Can you work these out from the drawing? Everything is in mm from the part's minimum corner. Round coordinates to 2 decimals unless told otherwise and drop trailing zeros. Order: outer loops, then holes, each group sorted by start corner. A loop starts at its lowest first (then second) coordinate and runs counter-clockwise, first axis right, second up. Notation, with made-up numbers: (14, 7) - (48, 7) arc R26 ccw to (48, 27) - close; hole circle Ø8 at (23.5, 77). An arc over 180 degrees is marked (long way). Answer as a JSON object with one key per item and string values.
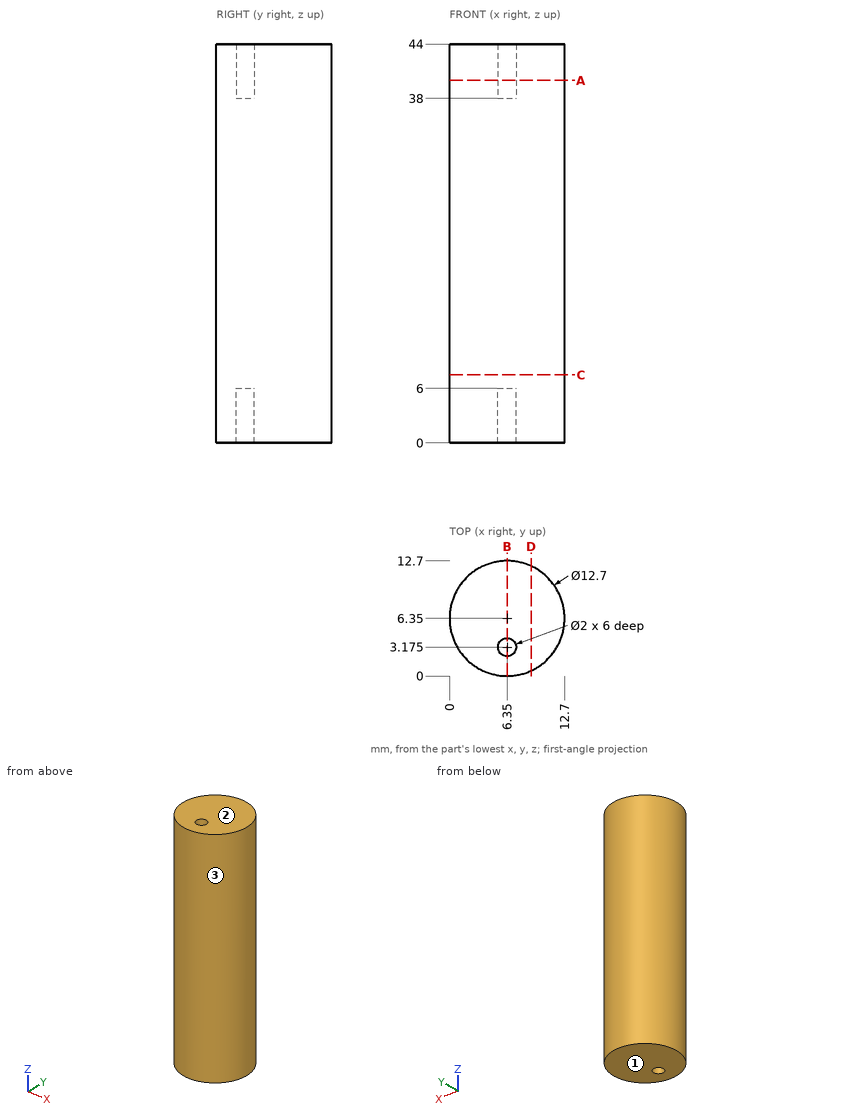
1. For P1, Ø1, axis at x = 9, y = 3.5, coming from the -Z side; P2, Ø6, axis at y = 11, z = 24, coming from the -X side; P3, Ø4, axis at x = 11.5, z = 36, coming from the +Y side; P4, Ø1.5, axis at x = 4.5, z = 31, coming from the +Y side, each with a flat end and sliding along its axis, tell me the tip position at first contact or that it passes through.
Responses:
{"P1": "z = 0", "P2": "x = 0.22", "P3": "y = 11.86", "P4": "y = 12.6"}
2. Thinking about a two-plate mould opening in Z: for the marked faces 1, 2 and 3, which applies, pulls with the +Z half, pulls with the -Z half, needs draft (parallel to the pull), parting line crosses it, or undercut?
Responses:
{"face 1": "pulls with the -Z half", "face 2": "pulls with the +Z half", "face 3": "needs draft"}
3. Imagine slicing it at A-A (z = 40). List the corners of the cut face in (x, y) for me (3 decimals), plus the area to 3 significant figures.
Responses:
{"outline": "circle Ø12.7 at (6.35, 6.35); hole circle Ø2 at (6.35, 3.175)", "area": "124 mm2"}
4. Imagine slicing it at D-D (x = 9). List the corners of the cut face in (y, z) for me.
Responses:
{"outline": "(0.58, 0) - (12.12, 0) - (12.12, 44) - (0.58, 44) - close"}
5. Imagine slicing it at B-B (x = 6.35). List the corners of the cut face in (y, z) for me (3 decimals), plus the area to 3 significant figures.
Responses:
{"outline": "(0, 0) - (2.175, 0) - (2.175, 6) - (4.175, 6) - (4.175, 0) - (12.7, 0) - (12.7, 44) - (4.175, 44) - (4.175, 38) - (2.175, 38) - (2.175, 44) - (0, 44) - close", "area": "535 mm2"}
6. Imagine slicing it at C-C (z = 7.5). List the corners of the cut face in (x, y) for me.
Responses:
{"outline": "circle Ø12.7 at (6.35, 6.35)"}
7. If I drill on L1, parallel to Y at x = 6.35, z = 3.65 (3 decimals); L2, parallel to X at y = 6.5, z = 8; L3, parallel to Y at x = 11.25, z = 10.5, over which ranges is the centre line in solid material (lowest first)? Write a range as [from, to].
Responses:
{"L1": "[0, 2.175], [4.175, 12.7]", "L2": "[0, 12.7]", "L3": "[2.31, 10.39]"}
